from build123d import *

# Parameters (mm, degrees)
SKETCH1_R                 = 50.8
BOSS_EXTRUDE1_DEPTH       = 30.48
F_1_14_TAPPED_HOLE1_D     = 23.8125
F_1_14_TAPPED_HOLE1_DEPTH = 15.24
F_1_14_TAPPED_HOLE1_TIP   = 7.153996745
SKETCH4_R                 = 43.18
SKETCH4_R_2               = 34.29
CUT_EXTRUDE1_DEPTH        = 5.08
FILLET1_R                 = 0.635


with BuildPart() as part:
    # Sketch1 → Boss-Extrude1 (new body)
    with BuildSketch(Plane(origin=(0, 0, 0), x_dir=(1, 0, 0), z_dir=(0, 1, 0))):
        with Locations(Location((0, 0, 0), (0, 0, 90))):
            Circle(SKETCH1_R)
    extrude(amount=BOSS_EXTRUDE1_DEPTH)

    # 1-14 Tapped Hole1
    with Locations(Plane(origin=(0, 0, 0), x_dir=(-1, 0, 0), z_dir=(0, -1, 0))):
        with Locations((0, 0)):
            Hole(F_1_14_TAPPED_HOLE1_D / 2, depth=F_1_14_TAPPED_HOLE1_DEPTH)
            with Locations((0, 0, -(F_1_14_TAPPED_HOLE1_DEPTH + F_1_14_TAPPED_HOLE1_TIP / 2))):  # 118° drill point
                Cone(0, F_1_14_TAPPED_HOLE1_D / 2, F_1_14_TAPPED_HOLE1_TIP, mode=Mode.SUBTRACT)

    # Sketch4 → Cut-Extrude1 (cut)
    with BuildSketch(Plane(origin=(0, 30.48, 0), x_dir=(1, 0, 0), z_dir=(0, 1, 0))):
        with Locations(Location((0, 0, 0), (0, 0, 270))):
            Circle(SKETCH4_R)
        with Locations(Location((0, 0, 0), (0, 0, 270))):
            Circle(SKETCH4_R_2, mode=Mode.SUBTRACT)
    extrude(amount=-CUT_EXTRUDE1_DEPTH, mode=Mode.SUBTRACT)

    # Fillet1
    fillet1_edges = [part.edges().sort_by_distance(p)[0] for p in [
        (0, 25.4, -43.18),
        (0, 25.4, -34.29),
    ]]
    fillet(fillet1_edges, radius=FILLET1_R)


solid = part.part
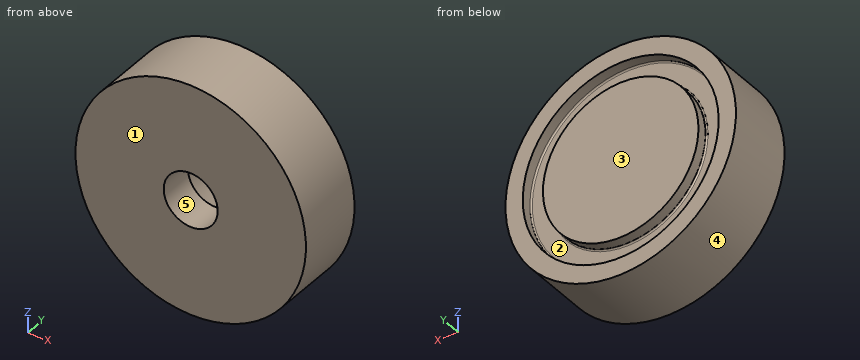
For this review, take the finished solid that the model builds, in its own axes (mm). Face numbers are marked on the shaded views. A direction names the side the tool comes from. Round coordinates to 2 decimals unless told otherwise and drop trailing zeros. Order: outer loops, then holes, each group sorted by start corner. A loop starts at its lowest first (then second) coordinate and runs counter-clockwise, first axis right, second up. Notation, with made-up numbers: (50.25, 36.25) -> (106.25, 36.25) arc R31 ccw to (106.25, 64.25) -> close; hole circle Ø7 at (29.25, 75.25). An arc over 180 degrees is marked (long way). Put each result on its own line as item: value.
Q1. Machinability: for the marked faces 1 and 2, which of the approach directions +Z, -Z, +X, -X, +Y, -Y give a long, thin tool a straight path to every point of the face, cutting with its end or side? Answer none if there is none.
Check result:
face 1: +Z, -Z, +X, -X, -Y
face 2: +Y
Q2. For probe 1 along X at (y, z) = (12, 0.5); probe 2 along Z at (x, y) = (2, 27.5); probe 3 along Y at (x, z) = (38.5, 17), list the stretches that pass through material, from the lowest coordinate up. Write a range as [from, to].
Check result:
probe 1: [-50.8, -11.9], [11.9, 50.8]
probe 2: [-50.76, -43.13], [-34.23, 34.23], [43.13, 50.76]
probe 3: [0, 25.4]
Q3. Insertion check: pin 1 Ø8 at (x, y) = (32.5, 20) entering from -Z; pin 2 Ø6 at (y, z) = (22.5, 7) entering from -X; pin 3 Ø5 at (x, z) = (0.5, -3.5) entering from -Y. Each pin has a flat end and moves straight along its axis. Give the tip position at first contact, or say it passes through.
Check result:
pin 1: z = -42.05
pin 2: x = -50.64
pin 3: y = 18.77
Q4. Mouldability with a two-part tool opening along X and no side actions: class the marked faces 3, 4 and 5 as pulls with the +X half, pulls with the -X half, needs draft (parallel to the pull), parting line crosses it, or undercut.
Check result:
face 3: needs draft
face 4: parting line crosses it
face 5: undercut
Q5. Add section A-A on y = 3.5. Write out the cut boundary in (x, z).
Check result:
outline: circle Ø101.6 at (0, 0); hole circle Ø23.81 at (0, 0)
